For this review, take the finished solid that the model builds, in its own axes (mm). Face numbers are marked on the shaded views. A direction names the side the tool comes from. Round coordinates to 2 decimals unless told otherwise and drop trailing zeros. Use one line per item in the form item = value. Start each with the question number.
from build123d import *

# Parameters (mm, degrees)
F0_W       = 45
F0_H       = 91
F0_R       = 14
F1_DEPTH   = 20
F3_R       = 7
F4_DEPTH   = 14
F7_DEPTH   = 16
F9_W       = 45
F9_H       = 43
F10_DEPTH  = 25
F12_R      = 7
F13_DEPTH  = 14
F13_FACE_R = 7
F14_DEPTH  = 15.248435


with BuildPart() as f1:
    # F0 (on Top) → F1 (new body)
    with BuildSketch(Plane.XY):
        with BuildLine():
            Line((-30.5, 14.547375), (-30.5, 45.5))
            Line((-30.5, 45.5), (-47.897288, 53.984803))
            ThreePointArc((-47.897288, 53.984803), (-43.595549, 50.111615), (-42, 44.547375))
            ThreePointArc((-42, 44.547375), (-47.84382, 35.136212), (-58.870473, 36.200695))
            Line((-58.870473, 36.200695), (-30.5, 14.547375))
        make_face()
        with BuildLine():
            ThreePointArc((-42, 44.547375), (-43.595549, 50.111615), (-47.897288, 53.984803))
            ThreePointArc((-47.897288, 53.984803), (-61.435875, 50.061007), (-58.870473, 36.200695))
            ThreePointArc((-58.870473, 36.200695), (-47.84382, 35.136212), (-42, 44.547375))
        make_face()
        Rectangle(F0_W, F0_H)
        with Locations((0, 15.5)):
            Circle(F0_R, mode=Mode.SUBTRACT)
        with BuildLine():
            Line((-22.5, -45.5), (-22.5, 45.5))
            Line((-22.5, 45.5), (-30.5, 45.5))
            Line((-30.5, 45.5), (-30.5, 14.547375))
            Line((-30.5, 14.547375), (-30.5, -29.491527))
            Line((-30.5, -29.491527), (-30.5, -33.539497))
            ThreePointArc((-30.5, -33.539497), (-25.61168, -35.564305), (-23.586872, -40.452625))
            ThreePointArc((-23.586872, -40.452625), (-25.026188, -44.675033), (-28.744805, -47.139226))
            Line((-28.744805, -47.139226), (-22.5, -45.5))
        make_face()
        with BuildLine():
            ThreePointArc((-35.864791, -36.092538), (-36.310734, -44.197851), (-28.744805, -47.139226))
            ThreePointArc((-28.744805, -47.139226), (-25.026188, -44.675033), (-23.586872, -40.452625))
            ThreePointArc((-23.586872, -40.452625), (-25.61168, -35.564305), (-30.5, -33.539497))
            ThreePointArc((-30.5, -33.539497), (-33.470648, -34.210302), (-35.864791, -36.092538))
        make_face()
        with BuildLine():
            Line((-30.5, -29.491527), (-35.864791, -36.092538))
            ThreePointArc((-35.864791, -36.092538), (-33.470648, -34.210302), (-30.5, -33.539497))
            Line((-30.5, -33.539497), (-30.5, -29.491527))
        make_face()
    extrude(amount=F1_DEPTH)

    # F3 (on face) → F4 (join)
    with BuildSketch(Plane(origin=(0, 42.452078, -11.375), x_dir=(1, 0, 0), z_dir=(0, -0.965926, 0.258819))):
        with BuildLine():
            ThreePointArc((-22.5, 46.776267), (0, 24.276267), (22.5, 46.776267))
            ThreePointArc((22.5, 46.776267), (0, 69.276267), (-22.5, 46.776267))
        make_face()
        with Locations((0, 46.776267)):
            Circle(F3_R, mode=Mode.SUBTRACT)
        with BuildLine():
            Line((22.5, 11.776267), (22.5, 46.776267))
            ThreePointArc((22.5, 46.776267), (0, 24.276267), (-22.5, 46.776267))
            Line((-22.5, 46.776267), (-22.5, 11.776267))
            Line((-22.5, 11.776267), (22.5, 11.776267))
        make_face()
        Polygon((90, 46.776267), (22.5, 46.776267), (22.5, 11.776267), (40, 11.776267), align=None)
    extrude(amount=F4_DEPTH)

    # F6 (on face) → F7 (join)
    with BuildSketch(Plane(origin=(0, 57.763138, 26.935393), x_dir=(-1, 0, 0), z_dir=(0, 0.906308, 0.422618))):
        with BuildLine():
            ThreePointArc((-78.482193, 42.09701), (-75.954981, 37.634972), (-75.078428, 32.582425))
            ThreePointArc((-75.078428, 32.582425), (-85.312715, 18.359627), (-102.050159, 23.544855))
            Line((-102.050159, 23.544855), (-90.000033, 7.582504))
            Line((-90.000033, 7.582504), (-22.441784, 7.582504))
            Line((-22.441784, 7.582504), (-78.482193, 42.09701))
        make_face()
        with BuildLine():
            ThreePointArc((-102.050159, 23.544855), (-85.312715, 18.359627), (-75.078428, 32.582425))
            ThreePointArc((-75.078428, 32.582425), (-75.954981, 37.634972), (-78.482193, 42.09701))
            ThreePointArc((-78.482193, 42.09701), (-99.356405, 44.368821), (-102.050159, 23.544855))
        make_face()
    extrude(amount=-F7_DEPTH)

    # F9 (on face) → F10 (join)
    with BuildSketch(Plane(origin=(0, -37.373418, -17.427511), x_dir=(1, 0, 0), z_dir=(0, -0.906308, -0.422618))):
        with Locations((0, 40.729131)):
            Rectangle(F9_W, F9_H)
    extrude(amount=-F10_DEPTH)

    # F12 (on face) → F13 (join)
    with BuildSketch(Plane(origin=(0, -69.15014, 18.528724), x_dir=(-1, 0, 0), z_dir=(0, 0.965926, -0.258819))):
        with BuildLine():
            ThreePointArc((-22.5, 46.163645), (0, 23.663645), (22.5, 46.163645))
            ThreePointArc((22.5, 46.163645), (0, 68.663645), (-22.5, 46.163645))
        make_face()
        with Locations((0, 46.163645)):
            Circle(F12_R, mode=Mode.SUBTRACT)
        with BuildLine():
            Line((22.5, 21.163645), (22.5, 46.163645))
            ThreePointArc((22.5, 46.163645), (0, 23.663645), (-22.5, 46.163645))
            Line((-22.5, 46.163645), (-22.5, 21.163645))
            Line((-22.5, 21.163645), (22.5, 21.163645))
        make_face()
    extrude(amount=F13_DEPTH)

    # F13_face (on face) → F14 (cut)
    with BuildSketch(Plane(origin=(0, -42.917516, 62.338362), x_dir=(-1, 0, 0), z_dir=(0, 0.965926, -0.258819))):
        with BuildLine():
            ThreePointArc((22.5, -2.942718), (0, 19.557282), (-22.5, -2.942718))
            Line((-22.5, -2.942718), (-22.5, -16.195324))
            Line((-22.5, -16.195324), (22.5, -16.195324))
            Line((22.5, -16.195324), (22.5, -2.942718))
        make_face()
        with Locations((0, -2.942718)):
            Circle(F13_FACE_R, mode=Mode.SUBTRACT)
    extrude(amount=F14_DEPTH, mode=Mode.SUBTRACT)


solid = f1.part
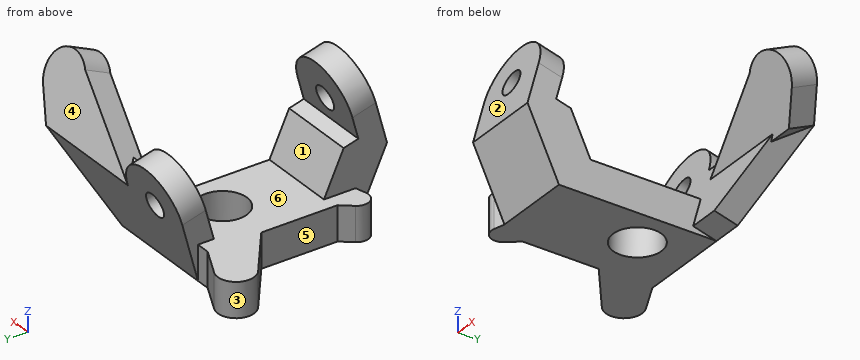
Item 1: Draft analysis for pull direction Y (two halves, no side actions). For the marked faces 1, 2 and 3, state which applies: +Y half, -Y half, draft (parallel to the pull), parting line (faces both ways), or undercut.
Item 2: Take a section at A-A on x = 0. Give the number of separate pieces and of enclosed holes in the cut face, plus the area to 3 significant figures.
Item 3: For P1, Ø10, axis at x = -4.5, z = 8, coming from the +Y side; P2, Ø22, axis at y = -14.5, z = 12.5, coming from the -X side; P3, Ø25, axis at x = 0, y = 15.5, coming from the -Z side; P4, Ø8, axis at x = 11.5, y = -1, coming from the -Z side, all flat-tipped, find the tip position at first contact; note any pin that passes through.
Item 4: Wall thickness on line 1 (Y direction, x = -9, z = 38); line 2 (X direction, y = 46.5, z = 41.5); line 3 (Y direction, x = 0, z = 4.25): over which ranges is each line inside the solid? List them lowest first.
Item 5: Machinability: for the marked faces 4, 5 and 6, which of the approach directions +Z, -Z, +X, -X, +Y, -Y give a long, thin tool a straight path to every point of the face, cutting with its end or side? Answer none if there is none.
Results:
q1.face_1 = undercut
q1.face_2 = -Y half
q1.face_3 = parting line
q2.separate_pieces = 4
q2.enclosed_holes = 0
q2.area = 2,790 mm2
q3.P1 = 48.98
q3.P2 = -30.5
q3.P3 = through
q3.P4 = 0
q4.line_1 = -63.22 to -35.64, 41.19 to 55.68
q4.line_2 = -21.86 to -4.52, 4.52 to 21.86, 39.29 to 97.83
q4.line_3 = -47.48 to 1.5, 29.5 to 46.64
q5.face_4 = +Z, +X, +Y
q5.face_5 = +Z, -Z, -X
q5.face_6 = +Z, -X
